Autodesk Inventor part; units mm, degrees
ref_plane "YZ Plane" through (0, 0, 0) normal (1, 0, 0) x (0, 1, 0)
ref_plane "XZ Plane" through (0, 0, 0) normal (0, 1, 0) x (-1, 0, 0)
ref_plane "XY Plane" through (0, 0, 0) normal (0, 0, 1) x (1, 0, 0)
sketch "Sketch1" plane through (0, 0, 0) normal (0, 0, 1) x (1, 0, 0)
  line L0 (0, 0) -> (68.9, 0)
  line L1 (68.9, 0) -> (68.9, 1.7)
  line L2 (68.9, 1.7) -> (0, 1.7)
  line L3 (0, 1.7) -> (0, 0)
  dimension "d0" = 68.9
  dimension "d1" = 1.7
extrude "Extrusion1" add sketch "Sketch1" along normal blind 53.3
sketch "Sketch2" plane through (0, 1.7, 0) normal (0, 1, 0) x (1, 0, 0)
  line L0 (0, -53.3) -> (68.9, -53.3)
  line L1 (68.9, 0) -> (68.9, -53.3)
  line L2 (68.9, 0) -> (0, 0)
  line L3 (0, 0) -> (0, -53.3)
  line L4 (66.2, 0) -> (66.2, -53.3)
  line L5 (68.9, -53.3) -> (0, -53.3)
  circle A0 centre (66.25, -47.55) radius 1.65
  circle A1 centre (66.25, -17.45) radius 1.65
  circle A2 centre (13.8, -2.65) radius 1.65
  circle A3 centre (13.95, -50.65) radius 1.65
  line L6 (66.2, 0) -> (66.2, -12.7)
  line L7 (66.2, -12.7) -> (68.9, -15.2036)
  line L8 (68.9, 0) -> (68.9, -15.2036)
  line L9 (68.9, 0) -> (68.9, -53.3)
  line L10 (66.2, 0) -> (68.9, 0)
  line L11 (0, 0) -> (68.9, 0)
  line L12 (68.9, 0) -> (66.2, 0)
  line L13 (66.2, -53.3) -> (66.2, -51.5)
  line L14 (66.2, -51.5) -> (68.9, -49.9641)
  line L15 (68.9, -53.3) -> (66.2, -53.3)
  line L16 (68.9, -53.3) -> (68.9, -49.9641)
  dimension "d4" = 2.7
  dimension "d5" = 5.75
  dimension "d6" = 1
  dimension "d7" = 3.3
  dimension "d8" = 3.3
  dimension "d9" = 3.3
  dimension "d10" = 3.3
  dimension "d11" = 15.8
  dimension "d12" = 1
  dimension "d13" = 1
  dimension "d14" = 1
  dimension "d15" = 13.8
  dimension "d16" = 12.3
  dimension "d17" = 12.7
  dimension "d18" = 2.5036
  dimension "d19" = 1.8
  dimension "d20" = 1.5359
extrude "Extrusion2" cut sketch "Sketch2" against normal blind 53.3 contours L4 L14 L1 L0 | L2 L1 L7 L4 | A0 L4 | L4 A0 | A1 L4 | L4 A1 | A2 | A3
sketch "Sketch3" plane through (0, 1.7, 53.3) normal (0, 1, 0) x (1, 0, 0)
  line L0 (66.2, 53.3) -> (0, 53.3)
  line L1 (0, 53.3) -> (0, 0)
  line L2 (0, 0) -> (66.2, 0)
  line L3 (9.75, 44.2) -> (-6.65, 44.2)
  line L4 (-6.65, 44.2) -> (-6.65, 32)
  line L5 (-6.65, 32) -> (9.75, 32)
  line L6 (9.75, 32) -> (9.75, 44.2)
  line L7 (12.3, 12.4) -> (-1.7, 12.4)
  line L8 (-1.7, 12.4) -> (-1.7, 3.6)
  line L9 (-1.7, 3.6) -> (12.3, 3.6)
  line L10 (12.3, 3.6) -> (12.3, 12.4)
  dimension "d23" = 9.1
  dimension "d24" = 9.75
  dimension "d25" = 16.4
  dimension "d26" = 12.2
  dimension "d27" = 8.8
  dimension "d28" = 14
  dimension "d29" = 12.4
  dimension "d30" = 1.7
extrude "Extrusion3" add sketch "Sketch3" along normal blind 10.8
sketch "Sketch4" plane through (0, 0, 0) normal (0, -1, 0) x (1, 0, 0)
  line L0 (1.7559, 51.8193) -> (11.7504, 51.8193)
  line L1 (11.7504, 51.8193) -> (11.7504, 41.2908)
  line L2 (11.7504, 41.2908) -> (1.7559, 41.2908)
  line L3 (1.7559, 41.2908) -> (1.7559, 51.8193)
  line L4 (2.8536, 9.1407) -> (9.75, 9.1407)
  line L5 (9.75, 9.1407) -> (9.75, 23.0608)
  line L6 (9.75, 23.0608) -> (2.8536, 23.0608)
  line L7 (2.8536, 23.0608) -> (2.8536, 9.1407)
  line L8 (17.3733, 1) -> (64.6, 1)
  line L9 (64.6, 1) -> (64.6, 3.3066)
  line L10 (64.6, 3.3066) -> (17.3733, 3.3066)
  line L11 (17.3733, 3.3066) -> (17.3733, 1)
  line L12 (14.8067, 10.5642) -> (19.5461, 10.5642)
  line L13 (19.5461, 10.5642) -> (19.5461, 5.2627)
  line L14 (19.5461, 5.2627) -> (14.8067, 5.2627)
  line L15 (14.8067, 5.2627) -> (14.8067, 10.5642)
  line L16 (23.3828, 51.8193) -> (64.9232, 51.8193)
  line L17 (64.9232, 51.8193) -> (64.9232, 49.9641)
  line L18 (64.9232, 49.9641) -> (23.3828, 49.9641)
  line L19 (23.3828, 49.9641) -> (23.3828, 51.8193)
  line L20 (63.5698, 43.7351) -> (27.6508, 43.7351)
  line L21 (27.6508, 43.7351) -> (27.6508, 41.2908)
  line L22 (27.6508, 41.2908) -> (63.5698, 41.2908)
  line L23 (63.5698, 41.2908) -> (63.5698, 43.7351)
  line L24 (63.5698, 37.8841) -> (27.6508, 37.8841)
  line L25 (27.6508, 37.8841) -> (27.6508, 35.2553)
  line L26 (27.6508, 35.2553) -> (63.5698, 35.2553)
  line L27 (63.5698, 35.2553) -> (63.5698, 37.8841)
  line L28 (63.1531, 29.6705) -> (67.0258, 29.6705)
  line L29 (67.0258, 29.6705) -> (67.0258, 20.8923)
  line L30 (67.0258, 20.8923) -> (63.1531, 20.8923)
  line L31 (63.1531, 20.8923) -> (63.1531, 29.6705)
extrude "Extrusion5" add sketch "Sketch4" along normal blind 1.2 contours L11 L10 L9 L8 | L12 L13 L14 L15 | L16 L17 L18 L19 | L23 L22 L21 L20 | L27 L26 L25 L24 | L28 L29 L30 L31
extrude "Extrusion6" add sketch "Sketch4" along normal blind 2.4 contours L0 L1 L2 L3 | L7 L6 L5 L4
sketch "Sketch5" plane through (0, 1.7, 0) normal (0, 1, 0) x (1, 0, 0)
  line L0 (16.8373, -1.3594) -> (65.158, -1.3594)
  line L1 (65.158, -1.3594) -> (65.158, -3.8941)
  line L2 (65.158, -3.8941) -> (16.8373, -3.8941)
  line L3 (16.8373, -3.8941) -> (16.8373, -1.3594)
  line L4 (14.3267, -5.2627) -> (19.5222, -5.2627)
  line L5 (19.5222, -5.2627) -> (19.5222, -8.6683)
  line L6 (19.5222, -8.6683) -> (14.3267, -8.6683)
  line L7 (14.3267, -8.6683) -> (14.3267, -5.2627)
  line L8 (67.0258, -29.6705) -> (67.0258, -20.8923)
  line L9 (63.1531, -20.8923) -> (67.0258, -20.8923)
  line L10 (67.0258, -20.8923) -> (67.0258, -28.4607)
  line L11 (67.0258, -28.4607) -> (63.1531, -28.4607)
  line L12 (63.1531, -28.4607) -> (63.1531, -20.8923)
  line L13 (23.3828, -52.3) -> (65.6017, -52.3)
  line L14 (65.6017, -52.3) -> (65.6017, -49.9641)
  line L15 (65.6017, -49.9641) -> (23.3828, -49.9641)
  line L16 (23.3828, -49.9641) -> (23.3828, -52.3)
  line L17 (27.2824, -35.2553) -> (63.9894, -35.2553)
  line L18 (63.9894, -35.2553) -> (63.9894, -44.4726)
  line L19 (63.9894, -44.4726) -> (27.2824, -44.4726)
  line L20 (27.2824, -44.4726) -> (27.2824, -35.2553)
  circle A0 centre (23.9092, -45.9) radius 2.5569
  circle A1 centre (18.2181, -45.9) radius 2.5569
extrude "Extrusion7" add sketch "Sketch5" along normal blind 8.4 contours L0 L1 L2 L3 | L4 L5 L6 L7 | L11 L12 L9 L8 | L16 L15 L14 L13 | L17 L18 L19 L20
extrude "Extrusion8" add sketch "Sketch5" along normal blind 5.6 contours A0 | A1
properties part number "Arduino"
Can you work these out from the model? Positions are in its coordinate system, mm. A direction names the side the tool comes from. Round coordinates to 2 decimals unless told otherwise and drop trailing zeros. Order: outer loops, then holes, each group sorted by start corner. A loop starts at its lowest first (then second) coordinate and runs counter-clockwise, first axis right, second up. Notation, with made-up numbers: (1, 81.25) -> (8, 81.25) arc R29 cw to (8, 118.25) -> close; hole circle Ø2 at (66.5, 58.25). An arc over 180 degrees is marked (long way). Write each question's results on one line, items separated by ' | '. Start each with the question number.
Item 1: If we section it at A-A, the plane y = 3.25: State how many separate pieces and enclosed holes the cut face has, then the cut area to 3 significant figures.
Item 2: Which directions (+Z, -Z, +X, -X, +Y, -Y) give clear straight access to the entire face, cutting with the end or side of a thin tool? Please do faces 5 (the flat face through (7, -1, 51.819)), 6 (the flat face through (5, 7, 40.9)), 7 (the flat face through (19.522, 6, 7)), 8 (the flat face through (66.2, 1, 52)).
Item 3: If we section it at B-B, the plane z = 17.45: Write out the boundary of the cut face in (x, y), then the cut area to 3 significant figures.
Item 4: If we section it at D-D, the plane z = 47.55: Write out the boundary of the cut face in (x, y).
Item 5: Please list where these lines run through material, in increasing order: L1, parallel to Z at x = 13.8, y = 1.05; L2, parallel to Z at x = 33, y = 2.5; L3, parallel to X at y = 1, z = 47.55.
Item 6: Thinking about a two-plate mould opening in X: for faces 1 (the cylindrical face through (14.84, 0.86, 49.26)), 2 (the flat face through (27.282, 6, 40)), 3 (the flat face through (7, -2.4, 47)), 4 (the flat face through (63.989, 6, 40)), which applies, +X half, -X half, draft (parallel to the pull), parting line (faces both ways), or undercut?
Item 7: Will these pins go through, and if not, where does the flat tip stop? pin 1 (1.3 mm diameter, centred on y = 6.5, z = 2.5, fed in from -X); pin 2 (2.5 mm diameter, centred on x = 24, z = 45, fed in from +Y); pin 3 (4 mm diameter, centred on x = 51.5, y = 5.5, fed in from +Z).
Results:
1) separate pieces: 9 | enclosed holes: 0 | area: 971 mm2
2) face 5: +Z, +X, -X, -Y | face 6: -X, +Y | face 7: +X, +Y | face 8: +Z, +X, +Y, -Y
3) outline: (-6.65, 1.7) -> (0, 1.7) -> (0, 0) -> (2.85, 0) -> (2.85, -2.4) -> (9.75, -2.4) -> (9.75, 0) -> (64.6, 0) -> (64.6, 1.7) -> (9.75, 1.7) -> (9.75, 12.5) -> (-6.65, 12.5) -> close; (67.9, 0) -> (68.9, 0) -> (68.9, 1.7) -> (67.9, 1.7) -> close | area: 305 mm2
4) outline: (-1.7, 1.7) -> (0, 1.7) -> (0, 0) -> (1.76, 0) -> (1.76, -2.4) -> (11.75, -2.4) -> (11.75, 0) -> (64.6, 0) -> (64.6, 1.7) -> (25.86, 1.7) -> (25.86, 7.3) -> (21.96, 7.3) -> (21.96, 1.7) -> (20.17, 1.7) -> (20.17, 7.3) -> (16.26, 7.3) -> (16.26, 1.7) -> (12.3, 1.7) -> (12.3, 12.5) -> (-1.7, 12.5) -> close; (67.9, 0) -> (68.9, 0) -> (68.9, 1.7) -> (67.9, 1.7) -> close
5) L1: z = 0 to 1, 4.3 to 49.01, 52.29 to 53.3 | L2: z = 1.36 to 3.89, 35.26 to 44.47, 49.96 to 52.3 | L3: x = 0 to 64.6, 67.9 to 68.9
6) face 1: undercut | face 2: undercut | face 3: draft | face 4: +X half
7) pin 1: stops at x = 16.84 | pin 2: stops at y = 7.3 | pin 3: stops at z = 52.3
